The model under review builds one solid part; all positions refer to its coordinate system, in mm. Face numbers are marked on the shaded views. A direction names the side the tool comes from. Round coordinates to 2 decimals unless told otherwise and drop trailing zeros. Loops run counter-clockwise (first coordinate to the right, second up) from the corner with the lowest first, then second, coordinate; pieces in that order, holes last. Notation, with made-up numbers: (50.25, 25) -> (108.25, 25) arc R23 ccw to (108.25, 49) -> close; hole circle Ø4 at (73, 3). An arc over 180 degrees is marked (long way). Use CSV: the item, a comma, the result in double quotes. Start each with the question number.
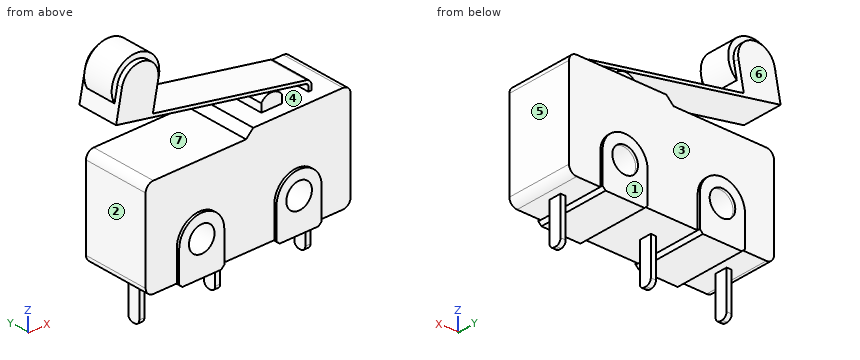
```python
from build123d import *

# Parameters (mm, degrees)
F0_R      = 1.25
F1_DEPTH  = 3.25
F2_R      = 1.25
F3_DEPTH  = 0.25
F4_R      = 1.25
F5_DEPTH  = 0.25
F6_R      = 0.75
F7_DEPTH  = 2
F8_W      = 3.4
F8_H      = 6
F9_DEPTH  = 25
F10_R     = 0.75
F11_DEPTH = 4
F12_W     = 0.5
F12_H     = 1.2
F13_DEPTH = 4.2
F14_R     = 0.5
F15_R     = 2.325
F15_R_2   = 0.8
F16_DEPTH = 1.5


with BuildPart() as f1:
    # F0 (on Front) → F1 (new body, symmetric)
    with BuildSketch(Plane.XZ):
        with BuildLine():
            ThreePointArc((0, 0.75), (0.2196699141, 0.2196699141), (0.75, 0))
            Line((0.75, 0), (3.05, 0))
            Line((3.05, 0), (3.35, -0.3))
            Line((3.35, -0.3), (7.15, -0.3))
            Line((7.15, -0.3), (7.45, 0))
            Line((7.45, 0), (12.55, 0))
            Line((12.55, 0), (12.85, -0.3))
            Line((12.85, -0.3), (16.65, -0.3))
            Line((16.65, -0.3), (16.95, 0))
            Line((16.95, 0), (19.25, 0))
            ThreePointArc((19.25, 0), (19.7803300859, 0.2196699141), (20, 0.75))
            Line((20, 0.75), (20, 9.45))
            ThreePointArc((20, 9.45), (19.7803300859, 9.9803300859), (19.25, 10.2))
            Line((19.25, 10.2), (10.5, 10.2))
            Line((10.5, 10.2), (9.8, 9.5))
            Line((9.8, 9.5), (0.75, 9.5))
            ThreePointArc((0.75, 9.5), (0.2196699141, 9.2803300859), (0, 8.75))
            Line((0, 8.75), (0, 0.75))
        make_face()
        with Locations((5.25, 3)):
            Circle(F0_R, mode=Mode.SUBTRACT)
        with Locations((14.75, 3)):
            Circle(F0_R, mode=Mode.SUBTRACT)
    extrude(amount=F1_DEPTH, both=True)

    # F2 (on face) → F3 (join)
    with BuildSketch(Plane.XZ.offset(3.25)):
        with BuildLine():
            Line((7.45, 0), (7.45, 3))
            ThreePointArc((7.45, 3), (5.25, 5.2), (3.05, 3))
            Line((3.05, 3), (3.05, 0))
            Line((3.05, 0), (3.35, -0.3))
            Line((3.35, -0.3), (7.15, -0.3))
            Line((7.15, -0.3), (7.45, 0))
        make_face()
        with Locations((5.25, 3)):
            Circle(F2_R, mode=Mode.SUBTRACT)
        with BuildLine():
            Line((16.95, 0), (16.95, 3))
            ThreePointArc((16.95, 3), (14.75, 5.2), (12.55, 3))
            Line((12.55, 3), (12.55, 0))
            Line((12.55, 0), (12.85, -0.3))
            Line((12.85, -0.3), (16.65, -0.3))
            Line((16.65, -0.3), (16.95, 0))
        make_face()
        with Locations((14.75, 3)):
            Circle(F2_R, mode=Mode.SUBTRACT)
    extrude(amount=F3_DEPTH)

    # F4 (on face) → F5 (join)
    with BuildSketch(Plane(origin=(0, 3.25, 0), x_dir=(-1, 0, 0), z_dir=(0, 1, 0))):
        with BuildLine():
            Line((-12.55, 0), (-12.55, 3))
            ThreePointArc((-12.55, 3), (-14.75, 5.2), (-16.95, 3))
            Line((-16.95, 3), (-16.95, 0))
            Line((-16.95, 0), (-16.65, -0.3))
            Line((-16.65, -0.3), (-12.85, -0.3))
            Line((-12.85, -0.3), (-12.55, 0))
        make_face()
        with Locations((-14.75, 3)):
            Circle(F4_R, mode=Mode.SUBTRACT)
        with BuildLine():
            Line((-3.05, 0), (-3.05, 3))
            ThreePointArc((-3.05, 3), (-5.25, 5.2), (-7.45, 3))
            Line((-7.45, 3), (-7.45, 0))
            Line((-7.45, 0), (-7.15, -0.3))
            Line((-7.15, -0.3), (-3.35, -0.3))
            Line((-3.35, -0.3), (-3.05, 0))
        make_face()
        with Locations((-5.25, 3)):
            Circle(F4_R, mode=Mode.SUBTRACT)
    extrude(amount=F5_DEPTH)

    # F6 (on Front) → F7 (join, symmetric)
    with BuildSketch(Plane.XZ):
        with BuildLine():
            Line((12.4, 10.2), (14.4, 10.2))
            Line((14.4, 10.2), (14.4, 11))
            ThreePointArc((14.4, 11), (13.4, 11.5366750419), (12.4, 11))
            Line((12.4, 11), (12.4, 10.2))
        make_face()
        with BuildLine():
            Line((17, 10.6529764402), (17, 10.2))
            Line((17, 10.2), (17.3, 10.2))
            Line((17.3, 10.2), (17.3, 10.6529764402))
            ThreePointArc((17.3, 10.6529764402), (17.1631848578, 11.0343683482), (16.8151340416, 11.2418262958))
            Line((16.8151340416, 11.2418262958), (1.8241165877, 14.1729239433))
            Line((1.8241165877, 14.1729239433), (2.3422197747, 16.8227482936))
            ThreePointArc((2.3422197747, 16.8227482936), (0.9210723325, 18.9346999851), (-1.1908793591, 17.5135525429))
            Line((-1.1908793591, 17.5135525429), (-1.7665495669, 14.5693032648))
            Line((-1.7665495669, 14.5693032648), (16.7575670208, 10.947401368))
            ThreePointArc((16.7575670208, 10.947401368), (16.9315924289, 10.8436723942), (17, 10.6529764402))
        make_face()
        with Locations((0.5756702078, 17.1681504183)):
            Circle(F6_R, mode=Mode.SUBTRACT)
    extrude(amount=F7_DEPTH, both=True)

    # F8 (on face) → F9 (cut)
    with BuildSketch(Plane(origin=(-4.4452524635, 0, 0.8691517489), x_dir=(0, -1, 0), z_dir=(-0.981416426, 0, 0.1918900693))):
        with Locations((0, 17.2595702214)):
            Rectangle(F8_W, F8_H)
    extrude(amount=F9_DEPTH, mode=Mode.SUBTRACT)

    # F12 (on face) → F13 (join)
    with BuildSketch(Plane(origin=(0, 0, 0), x_dir=(1, 0, 0), z_dir=(0, 0, -1))):
        with Locations((18.2, 0)):
            Rectangle(F12_W, F12_H)
        with Locations((9.4, 0)):
            Rectangle(F12_W, F12_H)
        with Locations((2, 0)):
            Rectangle(F12_W, F12_H)
    extrude(amount=F13_DEPTH)

    # F14
    f14_edges = [f1.edges().sort_by_distance(p)[0] for p in [
        (2, -0.6, -4.2),
        (2, 0.6, -4.2),
        (9.4, 0.6, -4.2),
        (9.4, -0.6, -4.2),
        (18.2, -0.6, -4.2),
        (18.2, 0.6, -4.2),
    ]]
    fillet(f14_edges, radius=F14_R)



with BuildPart() as f11:
    # F10 (on face) → F11 (new body)
    with BuildSketch(Plane.XZ.offset(2)):
        with Locations((0.5756702078, 17.1681504183)):
            Circle(F10_R)
    extrude(amount=-F11_DEPTH)


with BuildPart() as f1_1:
    add(f1.part)

    add(f11.part)  # F16 merges F11
    # F15 (on Front) → F16 (join, symmetric)
    with BuildSketch(Plane.XZ):
        with Locations((0.5733088478, 17.1697099968)):
            Circle(F15_R)
        with Locations((0.5733088478, 17.1697099968)):
            Circle(F15_R_2, mode=Mode.SUBTRACT)
        with Locations((0.5733088478, 17.1697099968)):
            Circle(F15_R_2)
    extrude(amount=F16_DEPTH, both=True)


solid = f1_1.part
```
1. The part is to be moulded in two halves that separate along X. For the marked faces 1, 2, 3 and 4, say which applies: pulls with the +X half, pulls with the -X half, needs draft (parallel to the pull), parting line crosses it, or undercut.
2. Take a section at B-B, the plane z = 8.25. Give the boundary of the cut face in (x, y).
3. Take a section at A-A, the plane x = 5.25. Give the boundary of the cut face in (y, z), then the cut area to 3 significant figures.
4. For the marked faces 5, 6 and 7, list the 3-axis set-ups (+Z, -Z, +X, -X, +Y, -Y) from which the entire face can be reached by the end or side of a thin tool; tool diameter is ignored.
5. For line 1 along X through (y, z) = (3.4, 3); line 2 along X through (y, z) = (1, 3); line 3 along Z through (x, y) = (5.25, 3.4), list the stretches that pass through material, from the lowest coordinate up. Write a range as from..to.
6. Clearance check with flat-ended pins moving along their axes: P1, Ø3, axis at x = 15.5, y = -1, coming from the -Z side; P2, Ø4.5, axis at x = 0.5, z = 18, coming from the -Y side; P3, Ø1, axis at y = 0, z = -2.5, coming from the +X side. State where each tip first meets the part, or that it passes through.
7. Take a section at C-C, the plane x = 14.75. Give the boundary of the cut face in (y, z).
Results:
1,face 1,"needs draft"
1,face 2,"pulls with the -X half"
1,face 3,"undercut"
1,face 4,"undercut"
2,outline,"(0, -3.25) -> (20, -3.25) -> (20, 3.25) -> (0, 3.25) -> close"
3,outline,"(-3.5, -0.3) -> (3.5, -0.3) -> (3.5, 1.75) -> (-3.5, 1.75) -> close; (-3.5, 4.25) -> (3.5, 4.25) -> (3.5, 5.2) -> (3.25, 5.2) -> (3.25, 9.5) -> (-3.25, 9.5) -> (-3.25, 5.2) -> (-3.5, 5.2) -> close; (-2, 13.2) -> (2, 13.2) -> (2, 13.5) -> (-2, 13.5) -> close"
3,area,"50.2 mm²"
4,face 5,"+Z, -Z, +X, +Y, -Y"
4,face 6,"+Z, +X, -X, +Y"
4,face 7,"-X, +Y, -Y"
5,line 1,"3.05..4, 6.5..7.45, 12.55..13.5, 16..16.95"
5,line 2,"0..4, 6.5..13.5, 16..20"
5,line 3,"-0.3..1.75, 4.25..5.2"
6,P1,"z = -0.3"
6,P2,"y = -2"
6,P3,"x = 18.45"
7,outline,"(-3.5, -0.3) -> (3.5, -0.3) -> (3.5, 1.75) -> (-3.5, 1.75) -> close; (-3.5, 4.25) -> (3.5, 4.25) -> (3.5, 5.2) -> (3.25, 5.2) -> (3.25, 10.2) -> (-3.25, 10.2) -> (-3.25, 5.2) -> (-3.5, 5.2) -> close; (-2, 11.34) -> (2, 11.34) -> (2, 11.65) -> (-2, 11.65) -> close"
